The model under review builds one solid part; all positions refer to its coordinate system, in mm. A direction names the side the tool comes from. Coordinates: 2 decimals unless noted, no trailing zeros. Loops run counter-clockwise (first coordinate to the right, second up) from the corner with the lowest first, then second, coordinate; pieces in that order, holes last. Notation, with made-up numbers: M 62,32.5 L 72,32.5 A21 ccw 72,51.5 Z; hole C 79.5,7 d3. An arc over 180 degrees is marked long. Write item = value, one per line. Start each with the question number.
Q1. We need section D-D on x = -12. Give the boundary of the cut face in (y, z).
Q2. We need section C-C on y = 4. Give the boundary of the cut face in (x, z), and give its area (3 significant figures).
Q3. For faces 1 (the face through (-40, 1, 5)), 2 (the face through (30, 3.2, 17)), 3 (the face through (-30, 1, 17)), list the 3-axis set-ups (+Z, -Z, +X, -X, +Y, -Y) from which the entire face can be reached by the end or side of a thin tool; tool diameter is ignored.
Q4. We need section A-A on x = 26.5. Give the boundary of the cut face in (y, z), and give its area (3 significant figures).
Q5. We need section B-B on z = 20.5. Give the boundary of the cut face in (x, y), and give its area (3 significant figures).
Q6. Wall thickness on probe 1 along X at (y, z) = (0.75, 5); probe 2 along X at (y, z) = (5.5, 22); probe 3 along Z at (x, y) = (28, 3.25): over which ranges is each line inside the solid? List them lowest first.
Q7. Mouldability with a two-part tool opening along Z and no side actions: class faces 4 (the face through (0.751, 0.507, -4.615)), 5 (the face through (10, 1, 17)), 6 (the face through (-9.86, 4.35, 22.84)), 7 (the face through (1, 0, 0)) as released by +Z, released by -Z, zero draft, split by the parting line, or undercut.
Q8. Clearance check with flat-ended pins moving along their axes: pin 1 Ø1 at (y, z) = (0, -10.5) entering from -X; pin 2 Ø1.5 at (x, z) = (-22.5, 10.5) entering from -Y; pin 3 Ø1.7 at (x, z) = (26.5, 17.5) entering from -Y. State where each tip first meets the part, or that it passes through.
from build123d import *

# Parameters (mm, degrees)
BOSS_EXTRUDE1_DEPTH = 1.5
BOSS_EXTRUDE2_DEPTH = 20
LPATTERN1_COUNT     = 2
LPATTERN1_PITCH     = 40
SKETCH6_R           = 2.5
CUT_EXTRUDE1_DEPTH  = 20
CHAMFER2_SIZE       = 0.5


with BuildPart() as part:
    # Sketch1 → Boss-Extrude1 (new body)
    with BuildSketch(Plane(origin=(0, 0, 0), x_dir=(1, 0, 0), z_dir=(0, 1, 0))):
        with BuildLine():
            Line((-30, 17), (30, 17))
            ThreePointArc((30, 17), (37.071067812, 14.071067812), (40, 7))
            Line((40, 7), (40, -17))
            Line((40, -17), (-40, -17))
            Line((-40, -17), (-40, 7))
            ThreePointArc((-40, 7), (-37.071067812, 14.071067812), (-30, 17))
        make_face()
    extrude(amount=BOSS_EXTRUDE1_DEPTH)

    # Sketch3 → Boss-Extrude2 (add)
    with BuildSketch(Plane(origin=(40, 0, 0), x_dir=(0, 0, -1), z_dir=(1, 0, 0))):
        with BuildLine():
            Line((-17, 0), (-17.907653586, 0))
            ThreePointArc((-17.907653586, 0), (-18.19052708, -0.040842773), (-18.450293899, -0.160034828))
            ThreePointArc((-18.450293899, -0.160034828), (-24.133848537, 5.112645111), (-16.620855154, 3.199825859))
            Line((-16.620855154, 3.199825859), (-18.120855154, 3.199825859))
            ThreePointArc((-18.120855154, 3.199825859), (-22.882198948, 4.265810965), (-19.02991455, 1.271378817))
            ThreePointArc((-19.02991455, 1.271378817), (-18.731636803, 1.441110731), (-18.393538309, 1.5))
            Line((-18.393538309, 1.5), (-17, 1.5))
            Line((-17, 1.5), (-17, 0))
        make_face()
    boss_extrude2 = extrude(amount=-BOSS_EXTRUDE2_DEPTH)

    # LPattern1: Boss-Extrude2 ×2
    with Locations(*[(-i * LPATTERN1_PITCH, 0, 0) for i in range(1, LPATTERN1_COUNT)]):
        add(boss_extrude2)

    # Sketch6 → Cut-Extrude1 (cut)
    with BuildSketch(Plane(origin=(0, 1.5, 0), x_dir=(1, 0, 0), z_dir=(0, 1, 0))):
        with Locations(Location((-28, -5, 0), (0, 0, 270))):
            Circle(SKETCH6_R)
        with Locations(Location((0, 7, 0), (0, 0, 270))):
            Circle(SKETCH6_R)
        with Locations(Location((26.5, -5, 0), (0, 0, 270))):
            Circle(SKETCH6_R)
    extrude(amount=-CUT_EXTRUDE1_DEPTH, mode=Mode.SUBTRACT)

    # Chamfer2
    chamfer2_edges = [part.edges().sort_by_distance(p)[0] for p in [
        (-28, 1.5, 2.5),
        (0, 1.5, -9.5),
        (26.5, 1.5, 2.5),
    ]]
    chamfer(chamfer2_edges, length=CHAMFER2_SIZE)


solid = part.part
Returned:
q1.outline = M -0.16,18.45 A1 cw 0,17.91 L 0,-17 L 1.5,-17 L 1.5,18.39 A1 ccw 1.27,19.03 A2.5 cw long 3.2,18.12 L 3.2,16.62 A4 ccw long Z
q2.outline = M -20,16.7 L 0,16.7 L 0,18.25 L -20,18.25 Z; M -20,22.99 L 0,22.99 L 0,24.54 L -20,24.54 Z; M 20,16.7 L 40,16.7 L 40,18.25 L 20,18.25 Z; M 20,22.99 L 40,22.99 L 40,24.54 L 20,24.54 Z
q2.area = 124 mm^2
q3.face_1 = +Z, -Z, -X, +Y, -Y
q3.face_2 = -Z, +X, -X
q3.face_3 = +Z, -X, +Y, -Y
q4.outline = M -0.16,18.45 A1 cw 0,17.91 L 0,7.5 L 1,7.5 L 1.5,8 L 1.5,18.39 A1 ccw 1.27,19.03 A2.5 cw long 3.2,18.12 L 3.2,16.62 A4 ccw long Z; M 0,-17 L 1.5,-17 L 1.5,2 L 1,2.5 L 0,2.5 Z
q4.area = 71.9 mm^2
q5.outline = M -20,-0.8 L 0,-0.8 L 0,0.7 L -20,0.7 Z; M -20,5.7 L 0,5.7 L 0,7.2 L -20,7.2 Z; M 20,-0.8 L 40,-0.8 L 40,0.7 L 20,0.7 Z; M 20,5.7 L 40,5.7 L 40,7.2 L 20,7.2 Z
q5.area = 120 mm^2
q6.probe_1 = -40 to -30.5, -25.5 to 24, 29 to 40
q6.probe_2 = -20 to 0, 20 to 40
q6.probe_3 = 16.62 to 18.12, 23.12 to 24.62
q7.face_4 = undercut
q7.face_5 = released by +Z
q7.face_6 = undercut
q7.face_7 = zero draft
q8.pin_1 = -39.54
q8.pin_2 = 0
q8.pin_3 = -0.1
